Design review of the part built by this model. Coordinates are the model's own, in mm. Give positions to 0.01 mm unless a question says otherwise; leave off trailing zeros. Write each loop counter-clockwise with the first axis right and the second up, starting at its lowest first coordinate (ties: lowest second). Pieces come first, ordered by that corner, then holes. Notation, with made-up numbers: M -6,7 L 0,7 A16 ccw 0,12 Z; hole C 12.5,63.25 d1. An arc over 180 degrees is marked long. Use a Markdown table: item, result. Add a question column.
```python
from build123d import *

# Parameters (mm, degrees)
BOSS_EXTRUDE1_DEPTH = 5


with BuildPart() as part:
    # Sketch1 → Boss-Extrude1 (new body)
    with BuildSketch(Plane(origin=(0, 0, 0), x_dir=(1, 0, 0), z_dir=(0, 1, 0))):
        with BuildLine():
            ThreePointArc((-10, 88.436417838), (0, -89), (10, 88.436417838))
            Line((10, 88.436417838), (10, 135.723235147))
            ThreePointArc((10, 135.723235147), (0, 265.05), (-10, 135.723235147))
            Line((-10, 135.723235147), (-10, 88.436417838))
        make_face()
        with BuildLine():
            ThreePointArc((-7.55, 145.470191638), (-55.05, 200), (-7.55, 254.529808362))
            Line((-7.55, 254.529808362), (-7.55, 145.470191638))
        make_face(mode=Mode.SUBTRACT)
        with BuildLine():
            Line((7.55, 145.470191638), (7.55, 254.529808362))
            ThreePointArc((7.55, 254.529808362), (55.05, 200), (7.55, 145.470191638))
        make_face(mode=Mode.SUBTRACT)
        with BuildLine():
            Line((-78.377228836, -9.9), (78.377228836, -9.9))
            ThreePointArc((78.377228836, -9.9), (0, -79), (-78.377228836, -9.9))
        make_face(mode=Mode.SUBTRACT)
        with BuildLine():
            Line((78.377228836, 9.9), (-78.377228836, 9.9))
            ThreePointArc((-78.377228836, 9.9), (0, 79), (78.377228836, 9.9))
        make_face(mode=Mode.SUBTRACT)
    extrude(amount=BOSS_EXTRUDE1_DEPTH)


solid = part.part
```
(1) Add section A-A on x = 0. Give the boundary of the cut face in (y, z).
(2) Add section B-B on z = -200. Give the boundary of the cut face in (x, y).
(3) Add section D-D on z = 55. Give the boundary of the cut face in (x, y).
(4) Wall thickness on L1, parallel to X at y = 0.4, z = -191; L2, parallel to Z at x = -28.5, y = 3.15; L3, parallel to X at y = 2.7, z = -226: over which ranges is each line inside the solid? List them lowest first.
(5) For pin 1 (2 mm diameter, centred on x = -18, y = 1.5, fed in from +Z); pin 2 (1.5 mm diameter, centred on x = 13, y = 3, fed in from -Z); pin 3 (3 mm diameter, centred on y = 0.5, z = -111.5, fed in from +X), all flat-tipped, find the tip position at first contact; note any pin that passes through.
(6) The part is to be moulded in two halves that separate along Z. For faces 1 (the flat face through (0, 5, -89)), 2 (the cylindrical face through (-3.77, 2.46, 88.92)), say which applies: released by +Z, released by -Z, zero draft, split by the parting line, or undercut.
(7) Add section C-C on y = 2.7. Give the boundary of the cut face in (x, z), then the cut area to 3 significant figures.
From the geometry:
| question | item | result |
|---|---|---|
| 1 | outline | M 0,-265.05 L 5,-265.05 L 5,-79 L 0,-79 Z; M 0,-9.9 L 5,-9.9 L 5,9.9 L 0,9.9 Z; M 0,79 L 5,79 L 5,89 L 0,89 Z |
| 2 | outline | M -65.05,0 L -55.05,0 L -55.05,5 L -65.05,5 Z; M -7.55,0 L 7.55,0 L 7.55,5 L -7.55,5 Z; M 55.05,0 L 65.05,0 L 65.05,5 L 55.05,5 Z |
| 3 | outline | M -69.97,0 L -56.71,0 L -56.71,5 L -69.97,5 Z; M 56.71,0 L 69.97,0 L 69.97,5 L 56.71,5 Z |
| 4 | L1 | x = -64.42 to -54.31, -7.55 to 7.55, 54.31 to 64.42 |
| 4 | L2 | z = -258.47 to -247.1, -152.9 to -141.53, -84.31 to -73.68, -9.9 to 9.9, 73.68 to 84.31 |
| 4 | L3 | x = -59.63 to -48.52, -7.55 to 7.55, 48.52 to 59.63 |
| 5 | pin 1 | stops at z = 87.36 |
| 5 | pin 2 | stops at z = -263.89 |
| 5 | pin 3 | stops at x = 10 |
| 6 | face 1 | zero draft |
| 6 | face 2 | undercut |
| 7 | outline | M -10,-135.72 A65.05 ccw long 10,-135.72 L 10,-88.44 A89 ccw long -10,-88.44 Z; hole M -78.38,-9.9 A79 ccw 78.38,-9.9 Z; hole M -78.38,9.9 L 78.38,9.9 A79 ccw Z; hole M -7.55,-254.53 L -7.55,-145.47 A55.05 ccw Z; hole M 7.55,-254.53 A55.05 ccw 7.55,-145.47 Z |
| 7 | area | 14,800 mm^2 |
